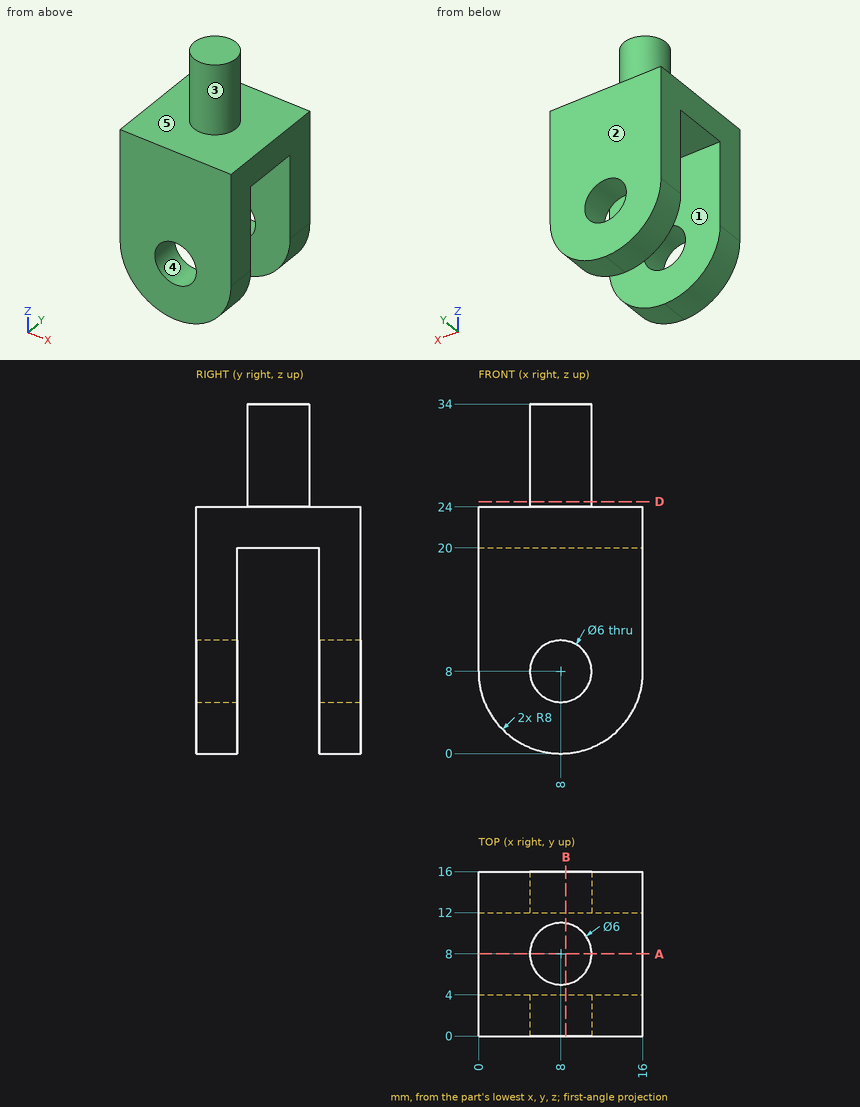
Source: three-view drawing plus pictorial views. Frame: mm from the lowest corner of the part. A direction names the side the tool comes from. Give positions to 0.01 mm unless a question says otherwise; leave off trailing zeros. Write each loop counter-clockwise with the first axis right and the second up, starting at its lowest first coordinate (ties: lowest second). Pieces come first, ordered by that corner, then holes. Notation, with made-up numbers: (-27, 61) - (8, 61) arc R24 cw to (8, 87) - close; hole circle Ø8 at (-4.5, 60.25). An arc over 180 degrees is marked (long way). Write item = value, one per line. Start each with the question number.
1. First-contact query: pin 1 Ø5.5 at (x, z) = (8, 8) entering from +Y; pin 2 Ø2.5 at (x, y) = (9.5, 7) entering from -Z. Flat tips, straight axial feed; report the tip coordinate or a pass-through.
2. Ray query, L1, parallel to Y at x = 6.25, z = 2.5; L2, parallel to X at y = 2, z = 8; L3, parallel to Z at x = 5.5, y = 6.75. Return the intervals inside material, ascending.
3. Access query for the marked faces 1 and 2. Directions: +Z, -Z, +X, -X, +Y, -Y. A direction counts if a zero-diameter tool reaches every point of the face in a straight line with its end or side. Return the directions, or none.
4. Section query D-D, the plane z = 24.5. Output: boundary loops of the cut face in (x, y), then the cut area to 3 significant figures.
5. Mould query, pull axis X, two halves, no side actions, for the marked faces 3, 4 and 5. Classes: released by +X, released by -X, zero draft, split by the parting line, or undercut.
6. Section query B-B, the plane x = 8.5. Output: boundary loops of the cut face in (y, z).
7. Section query A-A, the plane y = 8. Output: boundary loops of the cut face in (x, z), then the cut area to 3 significant figures.
Check sheet entries:
q1.pin_1 = through
q1.pin_2 = 20
q2.L1 = 0 to 4, 12 to 16
q2.L2 = 0 to 5, 11 to 16
q2.L3 = 20 to 34
q3.face_1 = -Z, +X, -X
q3.face_2 = +Z, -Z, +X, -X, +Y
q4.outline = circle Ø6 at (8, 8)
q4.area = 28.3 mm2
q5.face_3 = split by the parting line
q5.face_4 = undercut
q5.face_5 = zero draft
q6.outline = (0, 0.02) - (4, 0.02) - (4, 5.04) - (0, 5.04) - close; (0, 10.96) - (4, 10.96) - (4, 20) - (12, 20) - (12, 10.96) - (16, 10.96) - (16, 24) - (10.96, 24) - (10.96, 34) - (5.04, 34) - (5.04, 24) - (0, 24) - close; (12, 0.02) - (16, 0.02) - (16, 5.04) - (12, 5.04) - close
q7.outline = (0, 20) - (16, 20) - (16, 24) - (11, 24) - (11, 34) - (5, 34) - (5, 24) - (0, 24) - close
q7.area = 124 mm2
